Geometry check sheet. Reference: the model listing, model coordinates, mm. Coordinates: 2 decimals unless noted, no trailing zeros. Answer as a JSON object with one key per item and string values.
Autodesk Fusion 360 part; units mm, degrees
sketch "Sketch1" plane through (0, 0, 0) normal (0, 1, 0) x (1, 0, 0)
  line L0 (0, 0) -> (7.5, 0)
  line L1 (7.5, 0) -> (7.5, -6)
  line L2 (7.5, -6) -> (6.5, -6)
  line L3 (6.5, -6) -> (6.5, -7)
  line L4 (6.5, -7) -> (7.5, -7)
  line L5 (7.5, -7) -> (7.5, -10)
  line L6 (7.5, -10) -> (0, -10)
  line L7 (-7.5, -7) -> (-7.5, -10)
  line L8 (0, 0) -> (-7.5, 0)
  line L9 (-7.5, -6) -> (-6.5, -6)
  line L10 (-7.5, -10) -> (0, -10)
  line L11 (-7.5, 0) -> (-7.5, -6)
  line L12 (-6.5, -6) -> (-6.5, -7)
  line L13 (-6.5, -7) -> (-7.5, -7)
  dimension "d1" = 7.5
  dimension "d2" = 1
  dimension "d3" = 1
  dimension "d4" = 1
  dimension "d5" = 6
  dimension "d6" = 3
  dimension "d7" = 7.5
extrude "Extrude1" add sketch "Sketch1" along normal blind 700
sketch "Sketch2" plane through (0, 0, 10) normal (0, 0, 1) x (-1, 0, 0)
  line L0 (7.5, 0) -> (-7.5, 0)
  line L1 (-7.5, 0) -> (-7.5, -700)
  line L2 (-7.5, -700) -> (7.5, -700)
  line L3 (7.5, -700) -> (7.5, 0)
  circle A0 centre (0, -60) radius 2.25
  circle A1 centre (0, -126.6667) radius 2.25
  circle A2 centre (0, -193.3333) radius 2.25
  circle A3 centre (0, -260) radius 2.25
  circle A4 centre (0, -326.6667) radius 2.25
  circle A5 centre (0, -393.3333) radius 2.25
  circle A6 centre (0, -460) radius 2.25
  circle A7 centre (0, -526.6667) radius 2.25
  circle A8 centre (0, -593.3333) radius 2.25
  circle A9 centre (0, -660) radius 2.25
  dimension "d10" = 60
  dimension "d12" = 4.5
extrude "Extrude2" cut sketch "Sketch2" against normal up to surface (10 mm away) contours A0 | A1 | A2 | A3 | A4 | A5 | A6 | A7 | A8 | A9
sketch "Sketch3" plane through (0, 0, 10) normal (0, 0, 1) x (-1, 0, 0)
  circle A0 centre (0, -526.6667) radius 2.25
  circle A1 centre (0, -260) radius 2.25
  circle A2 centre (0, -60) radius 2.25
  circle A3 centre (0, -326.6667) radius 2.25
  circle A4 centre (0, -593.3333) radius 2.25
  circle A5 centre (0, -460) radius 2.25
  circle A6 centre (0, -193.3333) radius 2.25
  circle A7 centre (0, -126.6667) radius 2.25
  circle A8 centre (0, -393.3333) radius 2.25
  circle A9 centre (0, -660) radius 2.25
  line L0 (7.5, 0) -> (-7.5, 0)
  line L1 (-7.5, 0) -> (-7.5, -700)
  line L2 (-7.5, -700) -> (7.5, -700)
  line L3 (7.5, -700) -> (7.5, 0)
  circle A10 centre (0, -60) radius 3.75
  circle A11 centre (0, -126.6667) radius 3.75
  circle A12 centre (0, -193.3333) radius 3.75
  circle A13 centre (0, -260) radius 3.75
  circle A14 centre (0, -326.6667) radius 3.75
  circle A15 centre (0, -393.3333) radius 3.75
  circle A16 centre (0, -460) radius 3.75
  circle A17 centre (0, -526.6667) radius 3.75
  circle A18 centre (0, -593.3333) radius 3.75
  circle A19 centre (0, -660) radius 3.75
  dimension "d19" = 7.5
  dimension "d22" = 0
  dimension "d23" = -600
extrude "Extrude3" cut sketch "Sketch3" against normal blind 5.3 contours A10 | A11 | A12 | A13 | A14 | A15 | A16 | A17 | A18 | A19
1. Thickness scan on probe 1 along X at (y, z) = (60, 1.15); probe 2 along X at (y, z) = (660, 8.3); probe 3 along X at (y, z) = (406, 6.5). Record the ranges inside material, lowest first. Write a range as from..to.
Evaluation:
{"probe 1": "x = -7.5..-2.25, 2.25..7.5", "probe 2": "x = -7.5..-3.75, 3.75..7.5", "probe 3": "x = -6.5..6.5"}
2. Depth check by flat-ended pin: P1, Ø6, axis at x = 0, y = 326.67, coming from the -Z side; P2, Ø7, axis at x = 0, y = 526.67, coming from the +Z side; P3, Ø0.5, axis at y = 465, z = 6.5, coming from the +X side. Enter the tip coordinate at first touch or a pass-through.
Evaluation:
{"P1": "stops at z = 0", "P2": "stops at z = 4.7", "P3": "stops at x = 6.5"}
3. Section check A-A, the plane x = 0. State how many separate pieces and enclosed holes the cut face has, then the cut area to 3 significant figures.
Evaluation:
{"separate pieces": "11", "enclosed holes": "0", "area": "6,390 mm^2"}
